```python
from build123d import *

# Parameters (mm, degrees)
F0_W      = 40
F0_H      = 85
F1_DEPTH  = 1
F2_W      = 3
F2_H      = 3
F3_DEPTH  = 2
F5_DEPTH  = 3
F7_DEPTH  = 3
F9_R      = 1.5
F10_DEPTH = 45


with BuildPart() as f1:
    # F0 (on Top) → F1 (new body)
    with BuildSketch(Plane.XY):
        Rectangle(F0_W, F0_H)
    extrude(amount=F1_DEPTH)

    # F2 (on face) → F3 (join)
    with BuildSketch(Plane.XY.offset(1)):
        Polygon((-17, -42.5), (17, -42.5), (15.6843836329, -39.5), (-15.6843836329, -39.5), align=None)
        Polygon((-17, -39.5), (-17, -42.5), (-15.6843836329, -39.5), align=None)
        with Locations((-18.5, -41)):
            Rectangle(F2_W, F2_H)
        Polygon((15.6843836329, -39.5), (17, -42.5), (17, -39.5), align=None)
        with Locations((18.5, -41)):
            Rectangle(F2_W, F2_H)
        Polygon((17, -35.0301999523), (17, -39.5), (20, -39.5), (20, 39.5), (17, 39.5), (17, 35.0301999523), align=None)
        Polygon((15.6843836329, -39.5), (17, -39.5), (17, -35.0301999523), (1.6378985336, 0), (0, -3.7349000238), align=None)
        Polygon((-15.6843836329, -39.5), (0, -3.7349000238), (-1.6378985336, 0), (-17, -35.0301999523), (-17, -39.5), align=None)
        Polygon((-20, -39.5), (-17, -39.5), (-17, -35.0301999523), (-17, 35.0301999523), (-17, 39.5), (-20, 39.5), align=None)
        Polygon((-1.6378985336, 0), (0, -3.7349000238), (1.6378985336, 0), (0, 3.7349000238), align=None)
        Polygon((-17, 35.0301999523), (-1.6378985336, 0), (0, 3.7349000238), (-15.6843836329, 39.5), (-17, 39.5), align=None)
        Polygon((1.6378985336, 0), (17, 35.0301999523), (17, 39.5), (15.6843836329, 39.5), (0, 3.7349000238), align=None)
        with Locations((-18.5, 41)):
            Rectangle(F2_W, F2_H)
        Polygon((-17, 39.5), (-15.6843836329, 39.5), (-17, 42.5), align=None)
        Polygon((15.6843836329, 39.5), (17, 42.5), (-17, 42.5), (-15.6843836329, 39.5), align=None)
        Polygon((15.6843836329, 39.5), (17, 39.5), (17, 42.5), align=None)
        with Locations((18.5, 41)):
            Rectangle(F2_W, F2_H)
    extrude(amount=F3_DEPTH)

    # F4 (on face) → F5 (join)
    with BuildSketch(Plane.YZ.offset(20)):
        with BuildLine():
            ThreePointArc((-42.5, 3), (-42.2716385975, 4.1480502971), (-41.6213203436, 5.1213203436))
            Line((-41.6213203436, 5.1213203436), (-44.4490675498, 7.9490675498))
            ThreePointArc((-44.4490675498, 7.9490675498), (-46.5442111918, 7.0702264387), (-48.6547486938, 7.9114279791))
            Line((-48.6547486938, 7.9114279791), (-42.5, 1.7572743533))
            Line((-42.5, 1.7572743533), (-42.5, 3))
        make_face()
        with BuildLine():
            Line((-39.5, 3), (-36.5, 3))
            ThreePointArc((-36.5, 3), (-36.7387500509, 4.1728165749), (-37.4169991456, 5.1589598052))
            ThreePointArc((-37.4169991456, 5.1589598052), (-39.5268566208, 5.9998797846), (-41.6213203436, 5.1213203436))
            Line((-41.6213203436, 5.1213203436), (-39.5, 3))
        make_face()
        with BuildLine():
            Line((-42.5, 3), (-39.5, 3))
            Line((-39.5, 3), (-41.6213203436, 5.1213203436))
            ThreePointArc((-41.6213203436, 5.1213203436), (-42.2716385975, 4.1480502971), (-42.5, 3))
        make_face()
        with BuildLine():
            ThreePointArc((-37.4169991456, 5.1589598052), (-36.7387500509, 4.1728165749), (-36.5, 3))
            Line((-36.5, 3), (-35.1793104616, 3))
            Line((-35.1793104616, 3), (-37.4169991456, 5.1589598052))
        make_face()
        with BuildLine():
            ThreePointArc((-41.6213203436, 5.1213203436), (-39.5268566208, 5.9998797846), (-37.4169991456, 5.1589598052))
            Line((-37.4169991456, 5.1589598052), (-44.3843033436, 12.1262640032))
            ThreePointArc((-44.3843033436, 12.1262640032), (-43.7810708304, 11.1763673496), (-43.5701062619, 10.0710678119))
            ThreePointArc((-43.5701062619, 10.0710678119), (-43.798540858, 8.9226495455), (-44.4490675498, 7.9490675498))
            Line((-44.4490675498, 7.9490675498), (-41.6213203436, 5.1213203436))
        make_face()
        with BuildLine():
            ThreePointArc((-43.5701062619, 10.0710678119), (-43.7810708304, 11.1763673496), (-44.3843033436, 12.1262640032))
            Line((-44.3843033436, 12.1262640032), (-44.4121080066, 12.1540686663))
            Line((-44.4121080066, 12.1540686663), (-45.8270022514, 10.7391744215))
            ThreePointArc((-45.8270022514, 10.7391744215), (-45.6372408578, 10.4287928736), (-45.5710678119, 10.0710678119))
            ThreePointArc((-45.5710678119, 10.0710678119), (-45.6471882794, 9.6883843795), (-45.8639610307, 9.3639610307))
            Line((-45.8639610307, 9.3639610307), (-44.4490675498, 7.9490675498))
            ThreePointArc((-44.4490675498, 7.9490675498), (-43.798540858, 8.9226495455), (-43.5701062619, 10.0710678119))
        make_face()
        with BuildLine():
            ThreePointArc((-48.6547486938, 7.9114279791), (-46.5442111918, 7.0702264387), (-44.4490675498, 7.9490675498))
            Line((-44.4490675498, 7.9490675498), (-45.8639610307, 9.3639610307))
            ThreePointArc((-45.8639610307, 9.3639610307), (-46.5442025706, 9.0714287476), (-47.2391744215, 9.3270022514))
            Line((-47.2391744215, 9.3270022514), (-48.6547486938, 7.9114279791))
        make_face()
        with BuildLine():
            Line((-44.4121080066, 12.1540686663), (-44.3843033436, 12.1262640032))
            ThreePointArc((-44.3843033436, 12.1262640032), (-48.6791160167, 12.2069289943), (-48.6547486938, 7.9114279791))
            Line((-48.6547486938, 7.9114279791), (-47.2391744215, 9.3270022514))
            ThreePointArc((-47.2391744215, 9.3270022514), (-47.2781745931, 10.7781745931), (-45.8270022514, 10.7391744215))
            Line((-45.8270022514, 10.7391744215), (-44.4121080066, 12.1540686663))
        make_face()
    extrude(amount=-F5_DEPTH)

    # F6 (on face) → F7 (join)
    with BuildSketch(Plane(origin=(-20, 0, 0), x_dir=(0, -1, 0), z_dir=(-1, 0, 0))):
        with BuildLine():
            Line((36.5, 3), (42.5, 3))
            ThreePointArc((42.5, 3), (39.5, 6), (36.5, 3))
        make_face()
        with BuildLine():
            ThreePointArc((39.5000000598, 0), (41.6213203647, 0.8786796776), (42.5, 3))
            Line((42.5, 3), (36.5, 3))
            ThreePointArc((36.5, 3), (37.3786796776, 0.8786796353), (39.5000000598, 0))
        make_face()
    extrude(amount=-F7_DEPTH)

    # F8: union 

    # F9 (on face) → F10 (cut)
    with BuildSketch(Plane(origin=(-20, 0, 0), x_dir=(0, -1, 0), z_dir=(-1, 0, 0))):
        with Locations((39.5, 3)):
            Circle(F9_R)
    extrude(amount=-F10_DEPTH, mode=Mode.SUBTRACT)


solid = f1.part
```
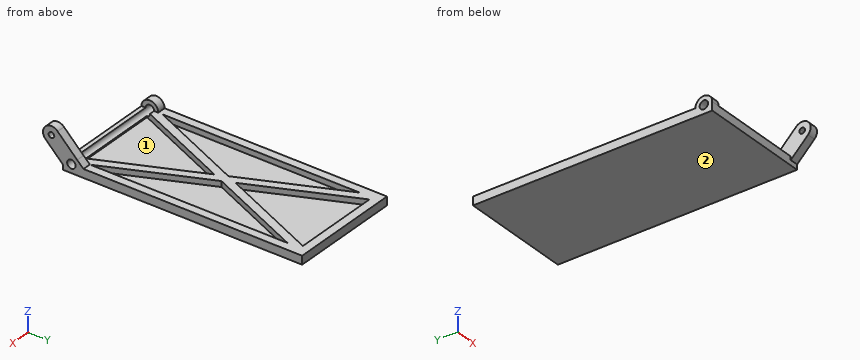
CAD build for the part. Positions are in the model's coordinates, mm. Face numbers are marked on the shaded views. Coordinates: 2 decimals unless noted, no trailing zeros. Write each loop counter-clockwise with the first axis right and the second up, starting at its lowest first coordinate (ties: lowest second). Pieces come first, ordered by that corner, then holes. Notation, with made-up numbers: (-37.5, 66.25) -> (-11.5, 66.25) arc R20 cw to (-11.5, 90.25) -> close; hole circle Ø10 at (-33.5, 35). An arc over 180 degrees is marked (long way). Return JSON: item names as keys, results as strings. Group by question number.
Q1. Cut at A-A, the plane x = 4. Give the cut face in (y, z).
Q2. Cut at C-C, the plane y = 23. Give the cut face in (x, z).
Q3. Flat gauge pins, fed straight in: pin 1 (7.5 mm diameter, centred on x = -7, y = 1, fed in from +Z); pin 2 (1.6 mm diameter, centred on x = -0.5, y = -41.5, fed in from +Z); pin 3 (2.5 mm diameter, centred on x = -4.5, z = 1.5, fed in from -Y). Where does each tip first touch, or does it go through?
Q4. Cut at B-B, the plane y = -1.5. Give the cut face in (x, z).
Q5. Drill centre lines: line 1 (X direction, y = 31, z = 1.75); line 2 (Y direction, x = 14, z = 1.25); line 3 (Y direction, x = -15, z = 2.5). Where is each one in solid material? Low to high.
Q6. Pull direction Y, two halves, no side cores. Call the marked faces 1 and 2: released by +Y, released by -Y, zero draft, split by the parting line, or undercut.
Returned:
{
 "1": {"outline": "(-42.5, 0) -> (42.5, 0) -> (42.5, 3) -> (39.5, 3) -> (39.5, 1) -> (12.86, 1) -> (12.86, 3) -> (5.39, 3) -> (5.39, 1) -> (-5.39, 1) -> (-5.39, 3) -> (-12.86, 3) -> (-12.86, 1) -> (-39.5, 1) -> (-39.5, 1.5) arc R1.5 cw to (-41, 3) -> (-42.5, 3) -> close"},
 "2": {"outline": "(-20, 0) -> (20, 0) -> (20, 3) -> (17, 3) -> (17, 1) -> (11.72, 1) -> (11.72, 3) -> (8.45, 3) -> (8.45, 1) -> (-8.45, 1) -> (-8.45, 3) -> (-11.72, 3) -> (-11.72, 1) -> (-17, 1) -> (-17, 3) -> (-20, 3) -> close"},
 "3": {"pin 1": "stops at z = 1", "pin 2": "stops at z = 3", "pin 3": "stops at y = -42.5"},
 "4": {"outline": "(-20, 0) -> (20, 0) -> (20, 3) -> (17, 3) -> (17, 1) -> (2.3, 1) -> (2.3, 3) -> (-2.3, 3) -> (-2.3, 1) -> (-17, 1) -> (-17, 3) -> (-20, 3) -> close"},
 "5": {"line 1": "x = -20 to -17, -15.23 to -11.96, 11.96 to 15.23, 17 to 20", "line 2": "y = -42.5 to -39.5, -35.66 to -28.19, 28.19 to 35.66, 39.5 to 42.5", "line 3": "y = -42.5 to -40.91, -37.94 to -30.47, 30.47 to 37.94, 39.5 to 42.5"},
 "6": {"face 1": "undercut", "face 2": "zero draft"}
}
